Here's how the part is built. I have some questions about the finished solid (model axes, mm). A direction names the side the tool comes from. Round coordinates to 2 decimals unless told otherwise and drop trailing zeros. Loops run counter-clockwise (first coordinate to the right, second up) from the corner with the lowest first, then second, coordinate; pieces in that order, holes last. Notation, with made-up numbers: M 78.25,-37.5 L 137.25,-37.5 A17 ccw 137.25,-28.5 Z; hole C 48,13 d8. An arc over 180 degrees is marked long. Write each question's results on one line, items separated by ' | '. Start each with the question number.
```python
from build123d import *

# Parameters (mm, degrees)
ESQUISSE1_W        = 73
ESQUISSE1_H        = 62.2
BOSS_EXTRU_1_DEPTH = 142
BOSS_EXTRU_2_START = -6
ESQUISSE2_R        = 16.5
BOSS_EXTRU_2_DEPTH = 61


with BuildPart() as part:
    # Esquisse1 → Boss.-Extru.1 (new body)
    with BuildSketch(Plane.XY):
        with Locations((36.5, 31.1)):
            Rectangle(ESQUISSE1_W, ESQUISSE1_H)
    extrude(amount=BOSS_EXTRU_1_DEPTH)

    # Esquisse2 → Boss.-Extru.2 (add)
    with BuildSketch(Plane(origin=(73, 0, 0), x_dir=(0, 0, -1), z_dir=(1, 0, 0)).offset(BOSS_EXTRU_2_START)):
        with Locations((-123.5, 49.6)):
            Circle(ESQUISSE2_R)
        with Locations((-88.5, 49.6)):
            Circle(ESQUISSE2_R)
        with Locations((-53.5, 49.6)):
            Circle(ESQUISSE2_R)
        with Locations((-18.5, 49.6)):
            Circle(ESQUISSE2_R)
        with Locations((-123.5, 12.6)):
            Circle(ESQUISSE2_R)
        with Locations((-88.5, 12.6)):
            Circle(ESQUISSE2_R)
        with Locations((-53.5, 12.6)):
            Circle(ESQUISSE2_R)
        with Locations((-18.5, 12.6)):
            Circle(ESQUISSE2_R)
    extrude(amount=-BOSS_EXTRU_2_DEPTH)


solid = part.part
```
1. For pin 1 (1.2 mm diameter, centred on y = -2.5, z = 22.5, fed in from +X); pin 2 (2 mm diameter, centred on y = -2, z = 58, fed in from -X), each with a flat end and sliding along its axis, tell me the tip position at first contact or that it passes through.
2. I want a section at A-A on x = 21. List the corners of the cut face in (y, z) for me.
3. I want a section at C-C on z = 116. List the corners of the cut face in (x, y) for me.
4. I want a section at B-B on z = 24. List the corners of the cut face in (x, y) for me, plus the area to 3 significant figures.
5. If we mould it in two halves opening along Z, with no side actions, what happens to faces 1 (the face through (36, 32, 0)), 2 (the face through (36, 32, 142)), 3 (the face through (36.9, -3.9, 53.7)), 4 (the face through (67, -1, 19))? For each: released by +Z, released by -Z, zero draft, split by the parting line, or undercut.
6. I want a section at D-D on z = 68. List the corners of the cut face in (x, y) for me.
7. Which directions (+Z, -Z, +X, -X, +Y, -Y) give clear straight access to the entire face, cutting with the end or side of a thin tool? Please do faces 5 (the face through (67, 64, 89)), 6 (the face through (67, -1, 89)), 7 (the face through (6, 64, 54)), 8 (the face through (6, -1, 19)).
8. I need wall thicknesses on line 1 along Y through (x, z) = (37, 7); line 2 along Z through (x, y) = (58.5, 63); line 3 along Y through (x, z) = (27.5, 28). Which ranges of each line are inside material? Lowest first, please.
Outcome:
1) pin 1: x = 67 | pin 2: x = 6
2) outline: M 0,0 L 62.2,0 L 62.2,7.85 A16.5 ccw 62.2,29.15 L 62.2,42.85 A16.5 ccw 62.2,64.15 L 62.2,77.85 A16.5 ccw 62.2,99.15 L 62.2,112.85 A16.5 ccw 62.2,134.15 L 62.2,142 L 0,142 L 0,134.15 A16.5 ccw 0,112.85 L 0,99.15 A16.5 ccw 0,77.85 L 0,64.15 A16.5 ccw 0,42.85 L 0,29.15 A16.5 ccw 0,7.85 Z
3) outline: M 0,0 L 6,0 L 6,-2.1 L 67,-2.1 L 67,0 L 73,0 L 73,62.2 L 67,62.2 L 67,64.3 L 6,64.3 L 6,62.2 L 0,62.2 Z
4) outline: M 0,0 L 6,0 L 6,-2.96 L 67,-2.96 L 67,0 L 73,0 L 73,62.2 L 67,62.2 L 67,65.16 L 6,65.16 L 6,62.2 L 0,62.2 Z | area: 4,900 mm2
5) face 1: released by -Z | face 2: released by +Z | face 3: undercut | face 4: zero draft
6) outline: M 0,0 L 73,0 L 73,62.2 L 0,62.2 Z
7) face 5: +Z, -Z, +X, +Y | face 6: +Z, -Z, +X, -Y | face 7: +Z, -Z, -X, +Y | face 8: +Z, -Z, -X, -Y
8) line 1: 0 to 62.2 | line 2: 8.87 to 28.13, 43.87 to 63.13, 78.87 to 98.13, 113.87 to 133.13 | line 3: -0.89 to 63.09
